Autodesk Fusion 360 part; units mm, degrees
sketch "Sketch1" plane through (0, 0, 0) normal (0, 0, 1) x (1, 0, 0)
  circle A0 centre (0, 0) radius 17.25
  circle A1 centre (0, 0) radius 15.75
  dimension "d1" = 34.5
  dimension "d4" = -1.5
ref_plane "WorkPlane1" through (0, 0, 20) normal (0, 0, 1) x (1, 0, 0)
sketch "Sketch2" plane through (0, 0, 20) normal (0, 0, 1) x (1, 0, 0)
  circle A0 centre (0, 0) radius 17.9
  circle A1 centre (0, 0) radius 16.4
  dimension "d3" = 35.8
  dimension "d5" = -1.5
ref_plane "WorkPlane2" through (0, 0, 35) normal (0, 0, 1) x (1, 0, 0)
sketch "Sketch3" plane through (0, 0, 35) normal (0, 0, 1) x (1, 0, 0)
  circle A0 centre (0, 0) radius 29.25
  circle A1 centre (0, 0) radius 31.25
  dimension "d7" = 58.5
  dimension "d8" = 2
loft "Loft1" add profiles "Sketch3", "Sketch2" section 1 section 2
loft "Loft2" cut profiles "Sketch3", "Sketch2" section 1 contours A0 section 2 contours A1
loft "Loft3" add profiles "Sketch2", "Sketch1" section 1 section 2
loft "Loft4" cut profiles "Sketch1", "Sketch2" section 1 contours A1 section 2 contours A1
extrude "Extrude1" add sketch "Sketch3" along normal blind 25
fillet "Fillet1" radius 15 2 edges at (-27.2706, 10.5773, 35) (-29.1352, 11.3005, 35)
fillet "Fillet2" radius 10 2 edges at (-16.6887, -6.4729, 20) (-15.2902, -5.9305, 20)
equation "d5 = d4"
Can you work these out from the model? Positions are in its coordinate system, mm. Round coordinates to 2 decimals unless told otherwise and drop trailing zeros. Loops run counter-clockwise (first coordinate to the right, second up) from the corner with the lowest first, then second, coordinate; pieces in that order, holes last.
Item 1: If we mould it in two halves opening along X, with no side actions, what happens to faces 1 (the conical face through (-13.903, -10.661, 8.305)), 2 (the flat face through (21, -21, 60)), 3 (the cylindrical face through (-6.341, 28.554, 50.137))? For each: +X half, -X half, draft (parallel to the pull), parting line (faces both ways), or undercut.
Item 2: Suppose I cut it at A-A, the plane z = 13. Write out the boundary of the cut face in (x, y) (1 decimal).
Item 3: Will these pins go through, and if not, where does the flat tip stop? pin 1 Ø1.5 at (y, z) = (9.5, 21.5) entering from -X; pin 2 Ø10 at (x, z) = (25, 31.5) entering from +Y; pin 3 Ø1.5 at (y, z) = (15, 49) entering from +X; pin 4 Ø2 at (x, y) = (-8, 14.5) entering from -Z.
Item 4: Please list where these lines run through material, in increasing order: L1, parallel to X at y = 0, z = 56; L2, parallel to X at y = -26, z = 39.5.
Reported:
1. face 1: parting line
1. face 2: draft
1. face 3: undercut
2. outline: circle Ø35.3 at (0, 0); hole circle Ø32.3 at (0, 0)
3. pin 1: stops at x = -17.63
3. pin 2: stops at y = 21.3
3. pin 3: stops at x = 27.81
3. pin 4: stops at z = 0
4. L1: x = -31.25 to -29.25, 29.25 to 31.25
4. L2: x = -17.25 to -13.32, 13.32 to 17.25
